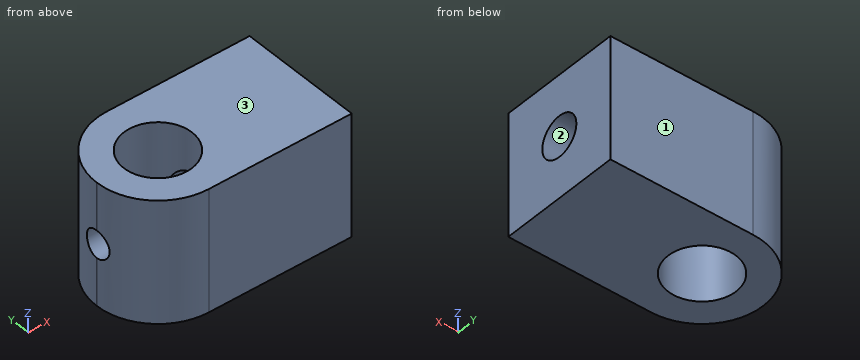
Solid Edge part; units mm, degrees
sketch "Sketch1" plane through (0, 0, 0) normal (0, -1, 0) x (1, 0, 0)
  line L0 (30, 18) -> (0, 18)
  line L1 (0, 18) -> (0, 0)
  line L2 (0, 0) -> (30, 0)
  line L3 (30, 0) -> (30, 18)
extrude "Protrusion1" add sketch "Sketch1" against normal blind 18
sketch "Sketch2" plane through (15, 9, 18) normal (0, 0, 1) x (1, 0, 0)
  circle A0 centre (-6, 0) radius 5
extrude "Recorte_Extrudado_1" cut sketch "Sketch2" against normal blind 18
fillet "Redondo_1" radius 9 2 edges at (0, 18, 9) (0, 0, 9)
extrude "Cutout1" [suppressed]
sketch "Sketch3" plane through (30, 9, 9) normal (1, 0, 0) x (0, 1, 0)
  circle A0 centre (0, 0) radius 3
extrude "Recorte_Extrudado_3" cut sketch "Sketch3" against normal blind 21
sketch "Sketch4" plane through (0, 0, 0) normal (-1, 0, 0) x (0, -1, 0)
  circle A0 centre (-9, 9) radius 2
extrude "Recorte_Extrudado_4" cut sketch "Sketch4" against normal blind 7
Verification items for the finished model (mm, model axes). Face numbers are marked on the shaded views. Round coordinates to 2 decimals unless told otherwise and drop trailing zeros. Write each loop counter-clockwise with the first axis right and the second up, starting at its lowest first coordinate (ties: lowest second). Pieces come first, ordered by that corner, then holes.
(1) Depth check by flat-ended pin: pin 1 Ø4 at (x, z) = (3.5, 6) entering from -Y; pin 2 Ø5 at (y, z) = (9, 9) entering from +X. Enter the tip coordinate at first touch or a pass-through.
Returned:
pin 1: stops at y = 0.71
pin 2: stops at x = 4.67
(2) Section check C-C (z = 9). Enter the section's corners in (x, y), plus the area to 3 significant figures.
Returned:
outline: (0.22, 7) arc R9 ccw to (9, 0) - (30, 0) - (30, 6) - (13, 6) arc R5 cw to (4.42, 7) - close; (0.22, 11) - (4.42, 11) arc R5 cw to (13, 12) - (30, 12) - (30, 18) - (9, 18) arc R9 ccw to start
area: 313 mm2
(3) Mould release check, pull along Z, two halves, no side actions. Record for the marked faces 1, 2 and 3: pulls with the +Z half, pulls with the -Z half, needs draft (parallel to the pull), parting line crosses it, or undercut.
Returned:
face 1: needs draft
face 2: undercut
face 3: pulls with the +Z half
(4) Material ranges on line 1 (Z direction, x = 2.4, y = 9); line 2 (Y direction, x = 9, z = 8.5); line 3 (X direction, y = 1.25, z = 4), recorded low to high.
Returned:
line 1: z = 0 to 7, 11 to 18
line 2: y = 0 to 4, 14 to 18
line 3: x = 4.42 to 30
(5) Section check A-A (y = 7.5). Enter the section's corners in (x, z), plus the area to 3 significant figures.
Returned:
outline: (0.13, 0) - (4.23, 0) - (4.23, 7.68) - (0.13, 7.68) - close; (0.13, 10.32) - (4.23, 10.32) - (4.23, 18) - (0.13, 18) - close; (13.77, 0) - (30, 0) - (30, 6.4) - (13.77, 6.4) - close; (13.77, 11.6) - (30, 11.6) - (30, 18) - (13.77, 18) - close
area: 271 mm2
(6) Section check B-B (x = 24.5). Enter the section's corners in (y, z), plus the area to 3 significant figures.
Returned:
outline: (0, 0) - (18, 0) - (18, 18) - (0, 18) - close; hole circle Ø6 at (9, 9)
area: 296 mm2
